```python
from build123d import *

# Parameters (mm, degrees)
F0_W     = 178
F0_H     = 17
F0_W_2   = 2.5
F0_H_2   = 13.5
F1_DEPTH = 15
F0_W_3   = 74
F2_DEPTH = 3


with BuildPart() as f1:
    # F0 (on Top) → F1 (new body)
    with BuildSketch(Plane.XY):
        Rectangle(F0_W, F0_H)
        Polygon((-10, -6.75), (-12.5, -6.75), (-86.5, -6.75), (-86.5, 6.75), (-12.5, 6.75), (-10, 6.75), (10, 6.75), (12.5, 6.75), (86.5, 6.75), (86.5, -6.75), (12.5, -6.75), (10, -6.75), align=None, mode=Mode.SUBTRACT)
        with Locations((-11.25, 0)):
            Rectangle(F0_W_2, F0_H_2)
        with Locations((11.25, 0)):
            Rectangle(F0_W_2, F0_H_2)
    extrude(amount=F1_DEPTH)

    # F0 (on Top) → F2 (join)
    with BuildSketch(Plane.XY):
        with Locations((-49.5, 0)):
            Rectangle(F0_W_3, F0_H_2)
        with Locations((49.5, 0)):
            Rectangle(F0_W_3, F0_H_2)
    extrude(amount=F2_DEPTH)


solid = f1.part
```
Here's how the part is built. I have some questions about the finished solid (model axes, mm). A direction names the side the tool comes from. Coordinates: 2 decimals unless noted, no trailing zeros. Order: outer loops, then holes, each group sorted by start corner. A loop starts at its lowest first (then second) coordinate and runs counter-clockwise, first axis right, second up.
1) Imagine slicing it at B-B on z = 9.75. List the corners of the cut face in (x, y) for me.
2) I need wall thicknesses on line 1 (X direction, y = 1.5, z = 4.25); line 2 (Y direction, x = 35, z = 8.5); line 3 (X direction, y = 3.75, z = 2). Which ranges of each line are inside material? Lowest first, please.
3) Will this pin go through, and if not, where does the flat tip stop? pin 1 (1.5 mm diameter, centred on x = -24, y = 0.5, fed in from +Z).
4) Imagine slicing it at C-C on x = -45.5. List the corners of the cut face in (y, z) for me, and give its area (3 significant figures).
5) Which directions (+Z, -Z, +X, -X, +Y, -Y) give clear straight access to the entire face, cutting with the end or side of a thin tool? Please do faces 1 (the face through (89, 0, 7)), 2 (the face through (-10, 0, 7)), 3 (the face through (-12.5, 0, 9)).
6) We'd pull the mould along Y, two halves only. Please class faces 4 (the face through (86.5, 0, 9)), 5 (the face through (0, 7, 15)), 6 (the face through (-1, -8.5, 7)): +Y half, -Y half, draft (parallel to the pull), parting line (faces both ways), or undercut.
7) Imagine slicing it at A-A on y = 2. List the corners of the cut face in (x, z) for me, and give its area (3 significant figures).
Response values:
1. outline: (-89, -8.5) - (89, -8.5) - (89, 8.5) - (-89, 8.5) - close; hole (-86.5, -6.75) - (-12.5, -6.75) - (-12.5, 6.75) - (-86.5, 6.75) - close; hole (-10, -6.75) - (10, -6.75) - (10, 6.75) - (-10, 6.75) - close; hole (12.5, -6.75) - (86.5, -6.75) - (86.5, 6.75) - (12.5, 6.75) - close
2. line 1: x = -89 to -86.5, -12.5 to -10, 10 to 12.5, 86.5 to 89
2. line 2: y = -8.5 to -6.75, 6.75 to 8.5
2. line 3: x = -89 to -10, 10 to 89
3. pin 1: stops at z = 3
4. outline: (-8.5, 0) - (8.5, 0) - (8.5, 15) - (6.75, 15) - (6.75, 3) - (-6.75, 3) - (-6.75, 15) - (-8.5, 15) - close
4. area: 93.0 mm2
5. face 1: +Z, -Z, +X, +Y, -Y
5. face 2: +Z, -Z
5. face 3: +Z
6. face 4: undercut
6. face 5: draft
6. face 6: -Y half
7. outline: (-89, 0) - (-10, 0) - (-10, 15) - (-12.5, 15) - (-12.5, 3) - (-86.5, 3) - (-86.5, 15) - (-89, 15) - close; (10, 0) - (89, 0) - (89, 15) - (86.5, 15) - (86.5, 3) - (12.5, 3) - (12.5, 15) - (10, 15) - close
7. area: 594 mm2
